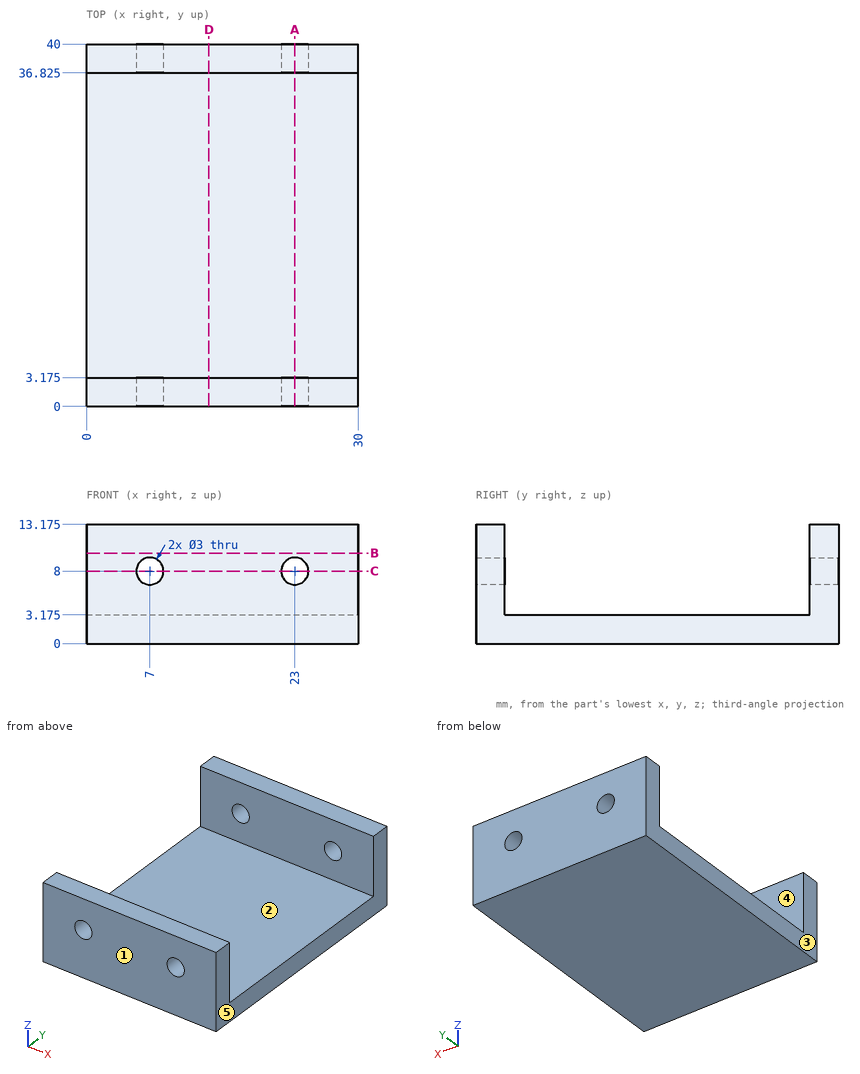
Study the drawing (mm; zero at the part's minimum x, y, z) and answer. A direction names the side the tool comes from. Round coordinates to 2 decimals unless told otherwise and drop trailing zeros. Loops run counter-clockwise (first coordinate to the right, second up) from the corner with the lowest first, then second, coordinate; pieces in that order, holes last.
Q1. For a pull along Y with two mould halves and no side action, classify the marked faces 1, 2 and 3 as released by +Y, released by -Y, zero draft, split by the parting line, or undercut.
Q2. Which of the six approach directions +Z, -Z, +X, -X, +Y, -Y give full straight-line access (tool end or side, diameter ignored) to the marked faces 4 and 5?
Q3. Section C-C, the plane z = 8 is taken. Determine the outline of the cut face in (x, y) (3 decimals).
Q4. Given pin 1 Ø1 at (x, y) = (8, 21.5) entering from +Z (3 decimals); pin 2 Ø2.5 at (x, z) = (23, 8) entering from +Y (3 decimals), each flat-ended and moving along its own axis, determine where each tip first touches the part or whether it passes through.
Q5. Section D-D, the plane x = 13.5 is taken. Determine the outline of the cut face in (y, z) (3 decimals), then the cut area to 4 significant figures.
Q6. Section A-A, the plane x = 23 is taken. Determine the outline of the cut face in (y, z) (3 decimals).
Q7. Find the intervals of material crossed by line 1 (X direction, y = 38.2, z = 8); line 2 (Y direction, x = 6.5, z = 3.5) (3 decimals); line 3 (Z direction, x = 7, y = 2.4) (3 decimals), in increasing order.
Q8. Section B-B, the plane z = 10 is taken. Determine the outline of the cut face in (x, y) (3 decimals).
Completed:
1. face 1: released by -Y
1. face 2: undercut
1. face 3: zero draft
2. face 4: +Z, +X, -X
2. face 5: +Z, -Z, +X, +Y, -Y
3. outline: (0, 0) - (5.5, 0) - (5.5, 3.175) - (0, 3.175) - close; (0, 36.825) - (5.5, 36.825) - (5.5, 40) - (0, 40) - close; (8.5, 0) - (21.5, 0) - (21.5, 3.175) - (8.5, 3.175) - close; (8.5, 36.825) - (21.5, 36.825) - (21.5, 40) - (8.5, 40) - close; (24.5, 0) - (30, 0) - (30, 3.175) - (24.5, 3.175) - close; (24.5, 36.825) - (30, 36.825) - (30, 40) - (24.5, 40) - close
4. pin 1: stops at z = 3.175
4. pin 2: passes through
5. outline: (0, 0) - (40, 0) - (40, 13.175) - (36.825, 13.175) - (36.825, 3.175) - (3.175, 3.175) - (3.175, 13.175) - (0, 13.175) - close
5. area: 190.5 mm2
6. outline: (0, 0) - (40, 0) - (40, 6.5) - (36.825, 6.5) - (36.825, 3.175) - (3.175, 3.175) - (3.175, 6.5) - (0, 6.5) - close; (0, 9.5) - (3.175, 9.5) - (3.175, 13.175) - (0, 13.175) - close; (36.825, 9.5) - (40, 9.5) - (40, 13.175) - (36.825, 13.175) - close
7. line 1: x = 0 to 5.5, 8.5 to 21.5, 24.5 to 30
7. line 2: y = 0 to 3.175, 36.825 to 40
7. line 3: z = 0 to 6.5, 9.5 to 13.175
8. outline: (0, 0) - (30, 0) - (30, 3.175) - (0, 3.175) - close; (0, 36.825) - (30, 36.825) - (30, 40) - (0, 40) - close
